The listing builds one solid part. Answer for the finished solid, in the listing's coordinates (mm). A direction names the side the tool comes from. Give positions to 0.01 mm unless a question says otherwise; leave off trailing zeros. Loops run counter-clockwise (first coordinate to the right, second up) from the corner with the lowest first, then second, coordinate; pieces in that order, holes last. Notation, with made-up numbers: M -17,41.25 L 36,41.25 A20 cw 36,60.25 Z; hole C -25.5,9 d5. An arc over 180 degrees is marked long. Return JSON: item names as keys, results as strings.
from build123d import *

# Parameters (mm, degrees)
F0_R        = 4.1
F1_DEPTH    = 15
F2_R        = 20
F3_DEPTH    = 70
F4_S5_R     = 4.1
F4_T6_DEPTH = 31


# Not quite as in the source:
# - a fillet or chamfer that OpenCascade refuses, or shapes differently, is made with other operations: its cross-section is extruded or revolved along the edge and cut away or added


with BuildPart() as f1:
    # F0 (on Top) → F1 (new body)
    with BuildSketch(Plane.XY):
        Circle(F0_R)
    extrude(amount=F1_DEPTH)

    # F2 (on Top) → F3 (join)
    with BuildSketch(Plane.XY):
        Circle(F2_R)
    extrude(amount=-F3_DEPTH)

    # F4: chamfer of 16 x 19.0680574815 on 1 edges, made by hand


with BuildPart() as f4_tool2:
    # F4_s3 → F4_t4 (revolve)
    with BuildSketch(Plane.XZ):
        Polygon((20, -19.0680574815), (4, 0), (20, 0), align=None)
    revolve(axis=Axis((0, 0, 0), (0, 0, 1)))

    # F4_s5 → F4_t6 (cut, symmetric)
    with BuildSketch(Plane.XY.offset(-9.5)):
        Circle(F4_S5_R)
    extrude(amount=F4_T6_DEPTH, both=True, mode=Mode.SUBTRACT)


with BuildPart() as f1_1:
    add(f1.part)

    # F4_t1: cut F4_tool2
    add(f4_tool2.part, mode=Mode.SUBTRACT)


solid = f1_1.part
(1) The part is cut by section A-A (x = 0). Determine the outline of the cut face in (y, z), and give its area (3 significant figures).
Values follow:
{"outline": "M -20,-70 L 20,-70 L 20,-19.07 L 4.1,-0.12 L 4.1,15 L -4.1,15 L -4.1,-0.12 L -20,-19.07 Z", "area": "2,620 mm²"}
(2) Determine the mould class of faces 3 (the flat face through (0, 0, 15)), 4 (the cylindrical face through (-4.336, -19.524, -44.178)) for opening direction Y: released by +Y, released by -Y, zero draft, split by the parting line, or undercut.
Values follow:
{"face 3": "zero draft", "face 4": "split by the parting line"}
(3) Given pin 1 (1.5 mm diameter, centred on y = 12.5, z = -59, fed in from +X); pin 2 (4 mm diameter, centred on x = -14, y = 10.5, fed in from +Z); pin 3 (6 mm diameter, centred on x = -13, y = -13.5, fed in from +Z), each flat-ended and moving along its own axis, determine where each tip first touches the part or whether it passes through.
Values follow:
{"pin 1": "x = 16.18", "pin 2": "z = -13.71", "pin 3": "z = -13.99"}
(4) The part is cut by section D-D (z = 1). Determine the outline of the cut face in (x, y), and give its area (3 significant figures).
Values follow:
{"outline": "C 0,0 d8.2", "area": "52.8 mm²"}
(5) A tool of negligible diameter and unlimited length cuts with its end or side. For faces 1 (the cylindrical face through (3.91, 1.23, 7.55)), 2 (the flat face through (0, 0, -70)), from which of +Z, -Z, +X, -X, +Y, -Y can it reach the whole face along a straight path? Write none if from no direction.
Values follow:
{"face 1": "+Z", "face 2": "-Z, +X, -X, +Y, -Y"}
(6) The part is cut by section C-C (z = -44.5). Determine the outline of the cut face in (x, y).
Values follow:
{"outline": "C 0,0 d40"}
(7) Straight lines are drawn through the part: line 1 along X through (y, z) = (0.5, -51.5); line 2 along Y through (x, z) = (-3, -25); line 3 along Y through (x, z) = (15, -38). For each, find the intervals that lie inside material, in ascending order.
Values follow:
{"line 1": "-19.99 to 19.99", "line 2": "-19.77 to 19.77", "line 3": "-13.23 to 13.23"}
